The listing builds one solid part. Answer for the finished solid, in the listing's coordinates (mm). Face numbers are marked on the shaded views. A direction names the side the tool comes from. Round coordinates to 2 decimals unless told otherwise and drop trailing zeros. Write each loop counter-clockwise with the first axis right and the second up, starting at its lowest first coordinate (ties: lowest second). Pieces come first, ordered by that corner, then holes. Notation, with made-up numbers: (20.5, 22) - (62.5, 22) arc R8 ccw to (62.5, 34) - close; hole circle Ø11 at (-2.75, 47.5). An arc over 180 degrees is marked (long way). Return JSON: item names as keys, results as strings. Group by question number.
(1) Section C-C, the plane y = -4 is taken. Write down the section's boundary in (x, z), then the cut area to 3 significant figures.
(2) Find the intervals of material crossed by line 1 along Y through (x, z) = (0, 0.2); line 2 along Z through (x, y) = (1.5, 4.75); line 3 along X through (y, z) = (5.74, 0.35), in increasing order. Write a range as [from, to].
(3) Section B-B, the plane y = 6 is taken. Write down the section's boundary in (x, z).
(4) This flat-tipped pin is pushed along its axis until it touches: pin 1 (5 mm diameter, centred on x = 4, y = 4, fed in from -Z). Where does it stop, or does it pass through?
(5) Section A-A, the plane y = 0 is taken. Write down the section's boundary in (x, z) (3 decimals), then the cut area to 3 significant figures.
(6) Which of the six approach directions +Z, -Z, +X, -X, +Y, -Y give full straight-line access (tool end or side, diameter ignored) to the marked faces 1 and 2?
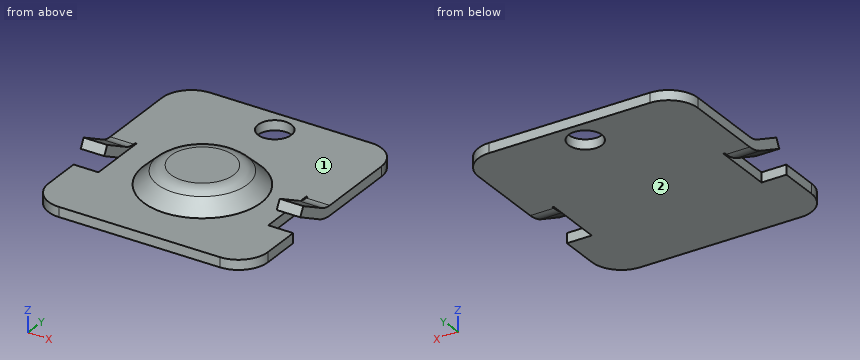
```python
from build123d import *

# Parameters (mm, degrees)
PAD_DEPTH     = 0.5
SKETCH001_R   = 0.76
HOLE_DEPTH    = 0.501
FILLET_R      = 1.5
SKETCH002_R   = 0.85
HOLE001_DEPTH = 0.501
PAD001_DEPTH  = 1.2
FILLET001_R   = 1


with BuildPart() as part:
    # Sketch → Pad (new body)
    with BuildSketch(Plane.XY):
        Polygon((0, -5), (5.6, -5), (5.6, -1.51), (4.33, -1.51), (4.33, 1.51), (5.6, 1.51), (5.6, 7), (1.5, 7), (-1.5, 7), (-5.6, 7), (-5.6, 1.51), (-4.33, 1.51), (-4.33, -1.51), (-5.6, -1.51), (-5.6, -5), align=None)
    extrude(amount=PAD_DEPTH)

    # Sketch001 → Hole (cut, through all)
    with BuildSketch(Plane.XY):
        with Locations((0, 11.84)):
            Circle(SKETCH001_R)
    extrude(amount=HOLE_DEPTH, mode=Mode.SUBTRACT)

    # Fillet
    fillet_edges = [part.edges().sort_by_distance(p)[0] for p in [
        (-5.6, 7, 0.25),
        (-5.6, -5, 0.25),
        (5.6, 7, 0.25),
        (5.6, -5, 0.25),
    ]]
    fillet(fillet_edges, radius=FILLET_R)

    # Sketch002 → Hole001 (cut, through all)
    with BuildSketch(Plane.XY):
        with Locations((0, 5.74)):
            Circle(SKETCH002_R)
    extrude(amount=HOLE001_DEPTH, mode=Mode.SUBTRACT)

    # Sketch003 → Revolution (revolve)
    with BuildSketch(Plane.YZ):
        Polygon((-3, 0.5), (0, 0.5), (0, 1.45), (-2, 1.45), align=None)
    revolve(axis=Axis((0, 0, 0), (0, 0, 1)))

    # Sketch004 → Pad001 (join)
    with BuildSketch(Plane.YZ.offset(5.6)):
        with BuildLine():
            Line((2, 0), (2, 0.5))
            Line((2, 0.5), (1.4, 0.5))
            ThreePointArc((0.790769, 0.651898), (1.086059, 0.538547), (1.4, 0.5))
            Line((0.790769, 0.651898), (-0.710242, 1.45))
            Line((-0.710242, 1.45), (-0.944978, 1.008526))
            Line((-0.944978, 1.008526), (0.556033, 0.210425))
            ThreePointArc((0.556033, 0.210425), (0.965098, 0.053399), (1.4, 0))
            Line((1.4, 0), (2, 0))
        make_face()
    pad001 = extrude(amount=-PAD001_DEPTH)

    # Fillet001
    fillet001_edges = [part.edges().sort_by_distance(p)[0] for p in [
        (0, 2, 1.45),
    ]]
    fillet(fillet001_edges, radius=FILLET001_R)

    # Mirrored: Pad001 across YZ
    add(pad001.mirror(Plane.YZ))


solid = part.part
```
Working result:
{
 "1": {"outline": "(-5.51, 0) - (5.51, 0) - (5.51, 0.5) - (-5.51, 0.5) - close", "area": "5.51 mm^2"},
 "2": {"line 1": "y = [-5, 4.89], [6.59, 7]", "line 2": "z = [0, 0.5]", "line 3": "x = [-5.58, -0.85], [0.85, 5.58]"},
 "3": {"outline": "(-5.51, 0) - (-0.81, 0) - (-0.81, 0.5) - (-5.51, 0.5) - close; (0.81, 0) - (5.51, 0) - (5.51, 0.5) - (0.81, 0.5) - close"},
 "4": {"pin 1": "stops at z = 0"},
 "5": {"outline": "(-5.6, 0.506) - (-4.4, 0.506) - (-4.4, 1.072) - (-5.6, 1.072) - close; (-4.33, 0) - (4.33, 0) - (4.33, 0.5) - (3, 0.5) - (2.289, 1.175) arc R1 ccw to (1.601, 1.45) - (-1.601, 1.45) arc R1 ccw to (-2.289, 1.175) - (-3, 0.5) - (-4.33, 0.5) - close; (4.4, 0.506) - (5.6, 0.506) - (5.6, 1.072) - (4.4, 1.072) - close", "area": "10.4 mm^2"},
 "6": {"face 1": "+Z", "face 2": "-Z, +X, -X, +Y, -Y"}
}
